Design review of the part built by this model. Coordinates are the model's own, in mm. Give positions to 0.01 mm unless a question says otherwise; leave off trailing zeros. Write each loop counter-clockwise with the first axis right and the second up, starting at its lowest first coordinate (ties: lowest second). Pieces come first, ordered by that corner, then holes. Notation, with made-up numbers: (-3.75, 84.25) -> (14.25, 84.25) arc R25 ccw to (14.25, 108.25) -> close; hole circle Ø11 at (-35.75, 59). An arc over 180 degrees is marked (long way). Answer as a JSON object with one key per item and string values.
```python
from build123d import *

# Parameters (mm, degrees)
SKETCH1_W                = 50.8
SKETCH1_H                = 50.8
SKETCH1_W_2              = 44.45
SKETCH1_H_2              = 44.45
BOSS_EXTRUDE1_DEPTH      = 590.55
BOSS_EXTRUDE1_DEPTH_BACK = 590.55
SKETCH6_W                = 50.8
SKETCH6_H                = 50.8
SKETCH6_W_2              = 44.45
SKETCH6_H_2              = 44.45
BOSS_EXTRUDE2_DEPTH      = 31.75
SKETCH7_R                = 21.082
CUT_EXTRUDE1_DEPTH       = 50.8


with BuildPart() as part:
    # Sketch1 → Boss-Extrude1 (new body, two sides)
    with BuildSketch(Plane(origin=(0, 0, 0), x_dir=(0, 0, -1), z_dir=(1, 0, 0))) as boss_extrude1_sk:
        Rectangle(SKETCH1_W, SKETCH1_H)
        Rectangle(SKETCH1_W_2, SKETCH1_H_2, mode=Mode.SUBTRACT)
    extrude(amount=BOSS_EXTRUDE1_DEPTH)
    extrude(boss_extrude1_sk.sketch, amount=-BOSS_EXTRUDE1_DEPTH_BACK)

    # Sketch6 → Boss-Extrude2 (add)
    with BuildSketch(Plane(origin=(590.55, 0, 0), x_dir=(0, 0, -1), z_dir=(1, 0, 0))):
        Rectangle(SKETCH6_W, SKETCH6_H)
        Rectangle(SKETCH6_W_2, SKETCH6_H_2, mode=Mode.SUBTRACT)
    extrude(amount=BOSS_EXTRUDE2_DEPTH)

    # Sketch7 → Cut-Extrude1 (cut)
    with BuildSketch(Plane(origin=(0, 25.4, 0), x_dir=(1, 0, 0), z_dir=(0, 1, 0))):
        with Locations((630.2375, 0)):
            Circle(SKETCH7_R)
    extrude(amount=-CUT_EXTRUDE1_DEPTH, mode=Mode.SUBTRACT)


solid = part.part
```
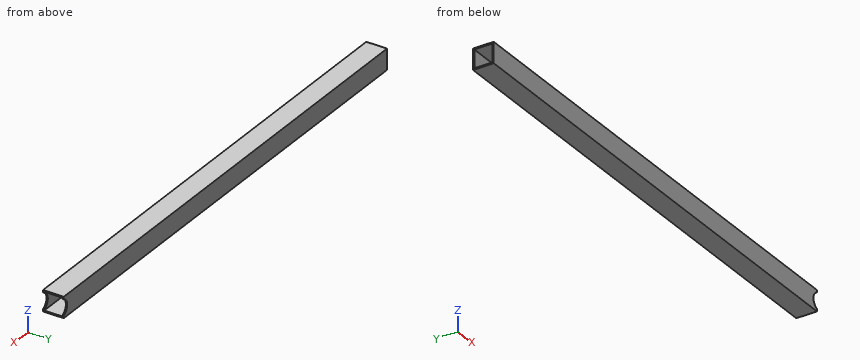
(1) We need section C-C, the plane z = 8.5. State the section outline as (x, y) points (3 decimals).
Here are the results:
{"outline": "(-590.55, -25.4) -> (610.945, -25.4) -> (610.945, -22.225) -> (-590.55, -22.225) -> close; (-590.55, 22.225) -> (610.945, 22.225) -> (610.945, 25.4) -> (-590.55, 25.4) -> close"}
(2) We need section A-A, the plane y = -9.5. State the section outline as (x, z) points (3 decimals).
Here are the results:
{"outline": "(-590.55, -25.4) -> (622.3, -25.4) -> (622.3, -22.225) -> (-590.55, -22.225) -> close; (-590.55, 22.225) -> (622.3, 22.225) -> (622.3, 25.4) -> (-590.55, 25.4) -> close"}
(3) We need section B-B, the plane x = 198.5. State the section outline as (y, z) points (3 decimals).
Here are the results:
{"outline": "(-25.4, -25.4) -> (25.4, -25.4) -> (25.4, 25.4) -> (-25.4, 25.4) -> close; hole (-22.225, -22.225) -> (22.225, -22.225) -> (22.225, 22.225) -> (-22.225, 22.225) -> close"}
(4) For line 1 along Y through (x, z) = (-301, -6) (3 decimals), list the stretches that pass through material, from the lowest coordinate up.
Here are the results:
{"line 1": "y = -25.4 to -22.225, 22.225 to 25.4"}
(5) Clearance check with a flat-ended pin moving along its axis: pin 1 (10 mm diameter, centred on y = 11, z = -14.5, fed in from +X) (3 decimals). State where the tip first meets the part, or that it passes through.
Here are the results:
{"pin 1": "passes through"}
